Answer from the drawing. Dimensions are ordinates in mm from the lowest x, y and z of the part. A direction names the side the tool comes from. Coordinates: 2 decimals unless noted, no trailing zeros. Loops run counter-clockwise (first coordinate to the right, second up) from the corner with the lowest first, then second, coordinate; pieces in that order, holes last.
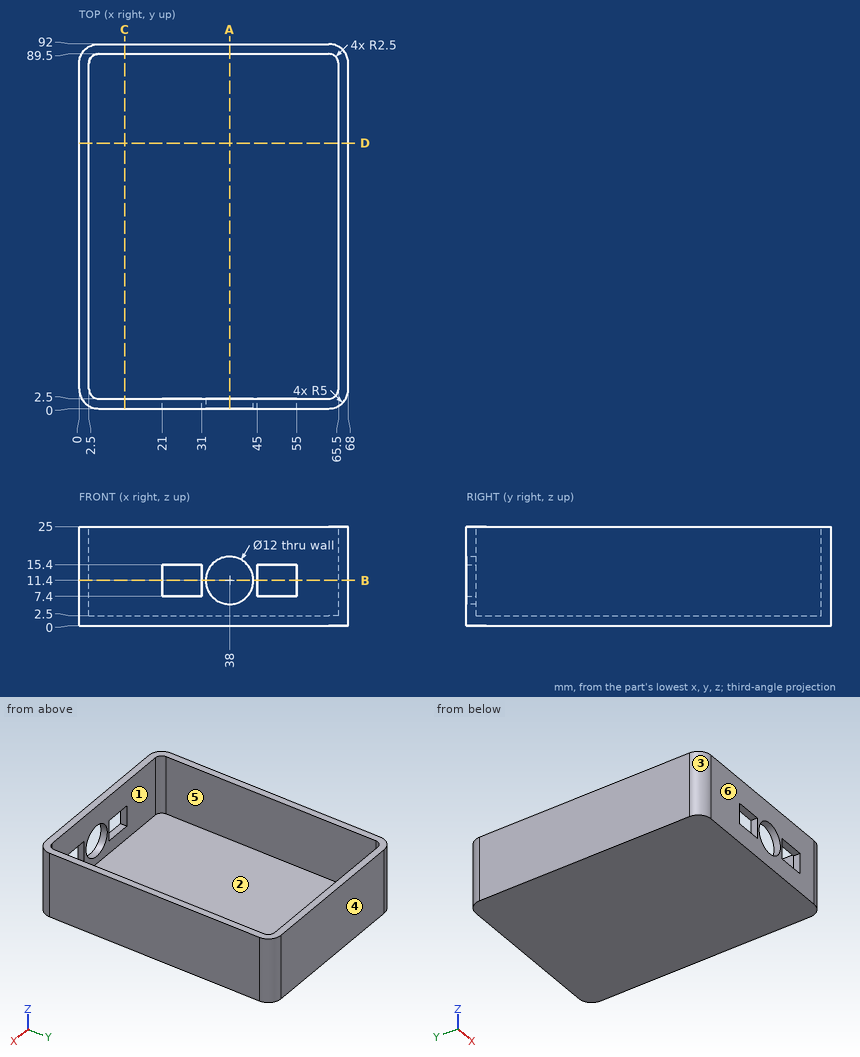
Item 1: A cutting plane is placed at B-B on z = 11.4. Determine the outline of the cut face in (x, y), then the cut area to 3 significant figures.
Numbers:
outline: (0, 5) arc R5 ccw to (5, 0) - (21, 0) - (21, 2.5) - (5, 2.5) arc R2.5 cw to (2.5, 5) - (2.5, 87) arc R2.5 cw to (5, 89.5) - (63, 89.5) arc R2.5 cw to (65.5, 87) - (65.5, 5) arc R2.5 cw to (63, 2.5) - (55, 2.5) - (55, 0) - (63, 0) arc R5 ccw to (68, 5) - (68, 87) arc R5 ccw to (63, 92) - (5, 92) arc R5 ccw to (0, 87) - close; (31, 0) - (32, 0) - (32, 2.5) - (31, 2.5) - close; (44, 0) - (45, 0) - (45, 2.5) - (44, 2.5) - close
area: 679 mm2
Item 2: A cutting plane is placed at D-D on y = 67. Determine the outline of the cut face in (x, z).
Numbers:
outline: (0, 0) - (68, 0) - (68, 25) - (65.5, 25) - (65.5, 2.5) - (2.5, 2.5) - (2.5, 25) - (0, 25) - close
Item 3: Determine the mould class of the marked faces 1, 2, 3 and 4 for opening direction X: released by +X, released by -X, zero draft, split by the parting line, or undercut.
Numbers:
face 1: undercut
face 2: undercut
face 3: released by -X
face 4: zero draft
Item 4: Find the intervals of material crossed by line 1 along X through (y, z) = (11, 4.5); line 2 along Y through (x, z) = (32, 20); line 3 along Z through (x, y) = (38, 2), in increasing order.
Numbers:
line 1: x = 0 to 2.5, 65.5 to 68
line 2: y = 0 to 2.5, 89.5 to 92
line 3: z = 0 to 5.4, 17.4 to 25
Item 5: Which of the six approach directions +Z, -Z, +X, -X, +Y, -Y give full straight-line access (tool end or side, diameter ignored) to the marked faces 5 and 6?
Numbers:
face 5: +Z
face 6: +Z, -Z, +X, -X, -Y
Item 6: Given pin 1 (1.2 mm diameter, centred on y = 1, z = 10, fed in from +X); pin 2 (9.5 mm diameter, centred on x = 38, z = 11.4, fed in from -Y); pin 3 (2.5 mm diameter, centred on y = 1.5, z = 13, fed in from +X), each flat-ended and moving along its own axis, determine where each tip first touches the part or whether it passes through.
Numbers:
pin 1: stops at x = 66.67
pin 2: stops at y = 89.5
pin 3: stops at x = 67.47
Item 7: A cutting plane is placed at C-C on x = 11.5. Determine the outline of the cut face in (y, z), then the cut area to 4 significant figures.
Numbers:
outline: (0, 0) - (92, 0) - (92, 25) - (89.5, 25) - (89.5, 2.5) - (2.5, 2.5) - (2.5, 25) - (0, 25) - close
area: 342.5 mm2
Item 8: A cutting plane is placed at A-A on x = 38. Determine the outline of the cut face in (y, z).
Numbers:
outline: (0, 0) - (92, 0) - (92, 25) - (89.5, 25) - (89.5, 2.5) - (2.5, 2.5) - (2.5, 5.4) - (0, 5.4) - close; (0, 17.4) - (2.5, 17.4) - (2.5, 25) - (0, 25) - close
